Part model, mm, in its own coordinate system. A direction names the side the tool comes from. Round coordinates to 2 decimals unless told otherwise and drop trailing zeros. Write each loop counter-clockwise with the first axis right and the second up, starting at its lowest first coordinate (ties: lowest second). Pieces come first, ordered by that corner, then holes. Notation, with made-up numbers: (59.25, -27.5) -> (88.25, -27.5) arc R35 ccw to (88.25, 8.5) -> close; hole circle Ø7 at (-27.75, 10.25). An arc over 180 degrees is marked (long way). Use CSV: the item, a comma, the result in double quotes. Start each with the question number.
(1) Saw through at B-B (x = -50.5). Give the cut face in (y, z), plus the area to 3 significant figures.
(2) Two-plate mould, pull along X, no slides. Class faces 6 (the flat face through (-20, -3, 3)), 7 (the flat face through (-70, -6, 3)), 8 (the flat face through (-40, -3, 3)), 9 (the flat face through (-60, -3, 3)): released by +X, released by -X, zero draft, split by the parting line, or undercut.
(3) Drop flat-ended pins along their axis: pin 1 (3 mm diameter, centred on y = -3.5, z = 2.5, fed in from -X); pin 2 (3 mm diameter, centred on x = -91, z = 2.5, fed in from -Y); pin 3 (1.8 mm diameter, centred on y = -1.5, z = 4, fed in from +X). Give the stop position or say it passes through.
(4) Saw through at A-A (z = 1.3). Give the cut face in (x, y).
(5) Which spindle directions (+Z, -Z, +X, -X, +Y, -Y) get a long thin tool onto all of the face, cutting with end or side? Do faces 1 (the flat face through (-10, 0, 3)), 2 (the flat face through (-80, -3, 3)), 3 (the flat face through (-50, 0, 3)), 4 (the flat face through (-100, 32, 3)), 5 (the flat face through (-51, 29, 0)). Say none if no direction does.
(6) Probe line 1 (X direction, y = -2, z = 3.9); line 2 (Y direction, x = -10.5, z = 2.35). List the from-to ranges inside material, lowest first. Write a range as [from, to].
```python
from build123d import *

# Parameters (mm, degrees)
ESQUISSE1_W        = 100
ESQUISSE1_H        = 64
BOSS_EXTRU_1_DEPTH = 6
ESQUISSE2_W        = 20
ESQUISSE2_H        = 6
BOSS_EXTRU_2_DEPTH = 6


with BuildPart() as part:
    # Esquisse1 → Boss.-Extru.1 (new body)
    with BuildSketch(Plane.XY):
        with Locations((-50, 32)):
            Rectangle(ESQUISSE1_W, ESQUISSE1_H)
    extrude(amount=BOSS_EXTRU_1_DEPTH)

    # Esquisse2 → Boss.-Extru.2 (add)
    with BuildSketch(Plane.XZ):
        with Locations((-70, 3)):
            Rectangle(ESQUISSE2_W, ESQUISSE2_H)
        with Locations((-30, 3)):
            Rectangle(ESQUISSE2_W, ESQUISSE2_H)
    extrude(amount=BOSS_EXTRU_2_DEPTH)


solid = part.part
```
Answers:
1,outline,"(0, 0) -> (64, 0) -> (64, 6) -> (0, 6) -> close"
1,area,"384 mm²"
2,face 6,"released by +X"
2,face 7,"zero draft"
2,face 8,"undercut"
2,face 9,"undercut"
3,pin 1,"stops at x = -80"
3,pin 2,"stops at y = 0"
3,pin 3,"stops at x = -20"
4,outline,"(-100, 0) -> (-80, 0) -> (-80, -6) -> (-60, -6) -> (-60, 0) -> (-40, 0) -> (-40, -6) -> (-20, -6) -> (-20, 0) -> (0, 0) -> (0, 64) -> (-100, 64) -> close"
5,face 1,"+Z, -Z, +X, -Y"
5,face 2,"+Z, -Z, -X, -Y"
5,face 3,"+Z, -Z, -Y"
5,face 4,"+Z, -Z, -X, +Y, -Y"
5,face 5,"-Z, +X, -X, +Y, -Y"
6,line 1,"x = [-80, -60], [-40, -20]"
6,line 2,"y = [0, 64]"
